For this review, take the finished solid that the model builds, in its own axes (mm). A direction names the side the tool comes from. Round coordinates to 2 decimals unless told otherwise and drop trailing zeros. Loops run counter-clockwise (first coordinate to the right, second up) from the corner with the lowest first, then second, coordinate; pieces in that order, holes last. Notation, with made-up numbers: M 87.25,11.5 L 121.25,11.5 A34 ccw 121.25,45.5 Z; hole C 64.5,-23.75 d1. An arc over 180 degrees is marked long. One line per question, with ' | ' between items. Start each with the question number.
1) We need section C-C (z = -11). Give the boundary of the cut face in (x, y).
2) We need section A-A (x = 0). Give the boundary of the cut face in (y, z).
3) We need section D-D (x = -41). Give the boundary of the cut face in (y, z), and give its area (3 significant figures).
4) For pin 1 Ø6.5 at (x, y) = (-19.05, 61) entering from -Z; pin 2 Ø19 at (x, y) = (-7.5, 20) entering from +Z; pin 3 Ø5 at (x, z) = (-23, 7.5) entering from +Y; pin 4 Ø13 at (y, z) = (24.5, -5) entering from +X, all flat-tipped, find the tip position at first contact; note any pin that passes through.
5) We need section B-B (y = -8). Give the boundary of the cut face in (x, z), and give its area (3 significant figures).
6) For probe 1 along Y at (x, z) = (0, -12); probe 2 along X at (y, z) = (2, 24.5); probe 3 along Z at (x, y) = (13.5, 68), list the stretches that pass through material, from the lowest coordinate up. Write a range as from..to.
7) Mouldability with a two-part tool opening along X and no side actions: class faces 4 (the face through (-26.9, 31.82, 20.27)), 5 (the face through (0.704, -31.992, 17.815)), 6 (the face through (-1.13, 69.82, -8.11)) as pulls with the +X half, pulls with the -X half, needs draft (parallel to the pull), parting line crosses it, or undercut.
8) For faces 1 (the face through (12.5, 25, -8)), 2 (the face through (-0.7, 84.18, -7.8)), 3 (the face through (-1, -36, -5)), list the 3-axis set-ups (+Z, -Z, +X, -X, +Y, -Y) from which the entire face can be reached by the end or side of a thin tool; tool diameter is ignored.
```python
from build123d import *

# Parameters (mm, degrees)
BOSS_EXTRUDE1_DEPTH          = 40
BOSS_EXTRUDE1_DEPTH_BACK     = 16
BOSS_EXTRUDE2_START          = -5
SKETCH1_3_R                  = 52.187837327
BOSS_EXTRUDE2_DEPTH          = 11
CUT_EXTRUDE1_DEPTH           = 57
CUT_EXTRUDE3_DEPTH           = 40
CUT_EXTRUDE4_DEPTH           = 85.187837327
FILLET1_R                    = 2
F_10_0_1935_DIAMETER_HOLE3_D = 4.9149
F_10_0_1935_DIAMETER_HOLE4_D = 4.9149
FILLET2_R                    = 2
FILLET3_R                    = 2


with BuildPart() as part:
    # Sketch1 → Boss-Extrude1 (new body, two sides)
    with BuildSketch(Plane.XY) as boss_extrude1_sk:
        with BuildLine():
            Line((-32, 0), (-32, 52.187837327))
            ThreePointArc((-32, 52.187837327), (0, 84.187837327), (32, 52.187837327))
            Line((32, 52.187837327), (32, 0))
            ThreePointArc((32, 0), (0, -32), (-32, 0))
        make_face()
    extrude(amount=BOSS_EXTRUDE1_DEPTH)
    extrude(boss_extrude1_sk.sketch, amount=-BOSS_EXTRUDE1_DEPTH_BACK)

    # Sketch1_3 → Boss-Extrude2 (add)
    with BuildSketch(Plane.XY.offset(BOSS_EXTRUDE2_START)):
        Circle(SKETCH1_3_R)
    extrude(amount=-BOSS_EXTRUDE2_DEPTH)

    # Sketch2 → Cut-Extrude1 (cut, through all)
    with BuildSketch(Plane.XY.offset(40)):
        with BuildLine():
            Line((-12.5, 0), (-12.5, 50))
            ThreePointArc((-12.5, 50), (0, 62.5), (12.5, 50))
            Line((12.5, 50), (12.5, 0))
            ThreePointArc((12.5, 0), (0, -12.5), (-12.5, 0))
        make_face()
    extrude(amount=-CUT_EXTRUDE1_DEPTH, mode=Mode.SUBTRACT)

    # Sketch6 → Cut-Extrude3 (cut)
    with BuildSketch(Plane.XY.offset(40)):
        with BuildLine():
            Line((-22, 0), (-22, 50))
            ThreePointArc((-22, 50), (0, 72), (22, 50))
            Line((22, 50), (22, 0))
            ThreePointArc((22, 0), (0, -22), (-22, 0))
        make_face()
    extrude(amount=-CUT_EXTRUDE3_DEPTH, mode=Mode.SUBTRACT)

    # Sketch7 → Cut-Extrude4 (cut, through all)
    with BuildSketch(Plane(origin=(32, 0, 0), x_dir=(0, 0, -1), z_dir=(1, 0, 0))):
        Polygon((0, 52.187837327), (0, 84.187837327), (-40, 84.187837327), (-40, 12), align=None)
    extrude(amount=-CUT_EXTRUDE4_DEPTH, mode=Mode.SUBTRACT)

    # Fillet1
    fillet1_edges = [part.edges().sort_by_distance(p)[0] for p in [
        (-27, 12, 40),
        (27, 12, 40),
    ]]
    fillet(fillet1_edges, radius=FILLET1_R)

    # 10 _0.1935_ Diameter Hole3 (through all)
    with Locations(Plane.XY):
        with Locations((-19.052558883, 61), (19.052558883, 61), (0, 72)):
            Hole(F_10_0_1935_DIAMETER_HOLE3_D / 2)

    # 10 _0.1935_ Diameter Hole4 (through all)
    with Locations(Plane(origin=(0, 0, -16), x_dir=(-1, 0, 0), z_dir=(0, 0, -1))):
        with Locations((0, -41), (41, 0), (-41, 0)):
            Hole(F_10_0_1935_DIAMETER_HOLE4_D / 2)

    # Fillet2
    fillet2_edges = [part.edges().sort_by_distance(p)[0] for p in [
        (-26.945471299, 52.187837327, 0),
        (26.945471299, 52.187837327, 0),
    ]]
    fillet(fillet2_edges, radius=FILLET2_R)

    # Fillet3
    fillet3_edges = [part.edges().sort_by_distance(p)[0] for p in [
        (-32, 41.225845835, -10.5),
        (32, 41.225845835, -10.5),
    ]]
    fillet(fillet3_edges, radius=FILLET3_R)


solid = part.part
```
Answers below:
1) outline: M -32.75,40.64 A52.19 ccw long 32.75,40.64 A2 cw 32,42.19 L 32,52.19 A32 ccw -32,52.19 L -32,42.19 A2 cw Z; hole C -41,0 d4.91; hole C -19.05,61 d4.91; hole M -12.5,0 A12.5 ccw 12.5,0 L 12.5,50 A12.5 ccw -12.5,50 Z; hole C 0,-41 d4.91; hole C 0,72 d4.91; hole C 19.05,61 d4.91; hole C 41,0 d4.91
2) outline: M -52.19,-16 L -43.46,-16 L -43.46,-5 L -52.19,-5 Z; M -38.54,-16 L -12.5,-16 L -12.5,0 L -22,0 L -22,40 L -32,40 L -32,-5 L -38.54,-5 Z; M 62.5,-16 L 69.54,-16 L 69.54,0 L 62.5,0 Z; M 74.46,-16 L 84.19,-16 L 84.19,0 L 74.46,0 Z
3) outline: M -32.29,-16 L -2.46,-16 L -2.46,-5 L -32.29,-5 Z; M 2.46,-16 L 32.29,-16 L 32.29,-5 L 2.46,-5 Z | area: 656 mm^2
4) pin 1: z = -16 | pin 2: z = 0 | pin 3: y = 47.16 | pin 4: x = 48.99
5) outline: M -51.57,-16 L -9.6,-16 L -9.6,0 L -20.49,0 L -20.49,40 L -30.98,40 L -30.98,-5 L -51.57,-5 Z; M 9.6,-16 L 51.57,-16 L 51.57,-5 L 30.98,-5 L 30.98,40 L 20.49,40 L 20.49,0 L 9.6,0 Z | area: 1,980 mm^2
6) probe 1: -52.19..-43.46, -38.54..-12.5, 62.5..69.54, 74.46..84.19 | probe 2: -32..-22, 22..32 | probe 3: -16..0
7) face 4: needs draft | face 5: parting line crosses it | face 6: undercut
8) face 1: +Z, -Z | face 2: +Z, -Z, +Y | face 3: +Z, -Y
